Source: CAD feature listing. Evaluate the final solid. Frame: model axes, mm. A direction names the side the tool comes from. Round coordinates to 2 decimals unless told otherwise and drop trailing zeros. Write each question's results on one line, items separated by ' | '. Start each with the question number.
1. Ray query, line 1 (Y direction, x = 0, z = -4.25) (3 decimals); line 2 (Y direction, x = 0, z = 15) (3 decimals); line 3 (X direction, y = 40.5, z = 4.5). Return the intervals inside material, ascending.
2. Section A-A on z = -14.5. Give the number of separate pieces and of enclosed holes in the cut face, and give its area (3 significant figures).
3. Draft query along X for faces 3 (the flat face through (-17, -51, -20.638)), 4 (the cylindrical face through (40.8, -18.1, 5.5)). Return one class per face: released by +X, released by -X, zero draft, split by the parting line, or undercut.
4. Set-up query: faces 1 (the cylindrical face through (-11.43, -51.45, 15.94)), 2 (the cylindrical face through (7.363, 43.945, 5.529)). Return all of +Z, -Z, +X, -X, +Y, -Y with unobstructed straight access to the full face (end or side cutting, diameter ignored); none if empty.
5. Contact query for flat-ended pins moving along their axis: pin 1 Ø5 at (x, z) = (16.5, -9.5) entering from +Y; pin 2 Ø10 at (x, y) = (35.5, -36.5) entering from -Z; pin 3 Ø3 at (x, z) = (-23.5, 7) entering from -Y. Output: stop coordinate, or through.
Autodesk Inventor part; units mm, degrees
ref_plane "Work Plane1" through (0, 0, 0) normal (0, 0, 1) x (1, 0, 0)
ref_plane "YZ Plane" through (0, 0, 0) normal (1, 0, 0) x (0, 1, 0)
ref_plane "XZ Plane" through (0, 0, 0) normal (0, 1, 0) x (-1, 0, 0)
sketch "Sketch1" plane through (0, 0, 0) normal (0, 0, 1) x (1, 0, 0)
  circle A0 centre (0, 0) radius 55.88
  circle A1 centre (0, 0) radius 9.525
  line L0 (7.391, 0) -> (3.6955, -6.4008)
  line L1 (3.6955, -6.4008) -> (-3.6955, -6.4008)
  line L2 (-3.6955, -6.4008) -> (-7.391, 0)
  line L3 (-7.391, 0) -> (-3.6955, 6.4008)
  line L4 (-3.6955, 6.4008) -> (3.6955, 6.4008)
  line L5 (3.6955, 6.4008) -> (7.391, 0)
  circle A2 centre (0, 0) radius 52.705
  point P0 (0, 9.525)
  dimension "d1" = 19.05
  dimension "d0" = 111.76
  dimension "d2" = 12.8016
  dimension "d3" = 3.175
extrude "Extrusion1" add sketch "Sketch1" along normal mid plane 41.275 contours A0 | A1 | A2
sketch "Sketch4" plane through (0, 0, 20.6375) normal (0, 0, 1) x (1, 0, 0)
  circle A0 centre (0, 0) radius 52.705
  circle A1 centre (0, 0) radius 55.88 construction
  dimension "d59" = 3.175
extrude "Extrusion4" cut sketch "Sketch4" against normal blind 12.7
sketch "Sketch5" plane through (0, 0, -20.6375) normal (0, 0, -1) x (-1, 0, 0)
  circle A0 centre (0, 0) radius 9.525
  line L0 (3.6955, 6.4008) -> (7.391, 0)
  line L1 (7.391, 0) -> (3.6955, -6.4008)
  line L2 (3.6955, -6.4008) -> (-3.6955, -6.4008)
  line L3 (-3.6955, -6.4008) -> (-7.391, 0)
  line L4 (-7.391, 0) -> (-3.6955, 6.4008)
  line L5 (-3.6955, 6.4008) -> (3.6955, 6.4008)
  line L6 (3.6955, 6.4008) -> (7.391, 0)
  dimension "d26" = 19.05
extrude "Extrusion5" add sketch "Sketch5" along normal blind 3.175
sketch "Sketch6" plane through (0, 0, -20.6375) normal (0, 0, -1) x (-1, 0, 0)
  circle A0 centre (0, 0) radius 52.705
  circle A1 centre (0, 0) radius 9.525
  circle A2 centre (0, 0) radius 55.88 construction
  dimension "d60" = 3.175
extrude "Extrusion6" cut sketch "Sketch6" against normal blind 23.8252
sketch "Sketch7" plane through (0, 0, 7.9375) normal (0, 0, 1) x (1, 0, 0)
  circle A0 centre (0, 0) radius 9.525
  circle A1 centre (0, 0) radius 52.705
  circle A2 centre (0, 0) radius 47.9425 construction
  circle A3 centre (0, 0) radius 14.2875 construction
  line L0 (-9.7714, 10.4237) -> (-9.7714, 46.9362) construction
  line L1 (-9.7714, 10.4237) -> (16.8454, 44.8856)
  line L2 (-9.7714, 10.4237) -> (-36.3881, 44.8856)
  arc A4 (16.8454, 44.8856) -> (-36.3881, 44.8856) centre (-9.7714, -126.8345) ccw
  point P0 (-6.5143, 6.9491)
  dimension "d42" = 4.7625
  dimension "d41" = 4.7625
  dimension "d43" = 34.4619
  dimension "d44" = 36.5125
  dimension "d45" = 4.7625
extrude "Extrusion8" [suppressed]
fillet "Fillet1" [suppressed]
pattern_circular "Circular Pattern1" [suppressed]
fillet "Fillet2" [suppressed]
sketch "Sketch8" plane through (0, 0, 20.6375) normal (0, 0, 1) x (1, 0, 0)
  circle A0 centre (0, 0) radius 55.88
  circle A1 centre (0, 0) radius 57.15
  dimension "d53" = 114.3
extrude "Extrusion9" add sketch "Sketch8" against normal blind 1.5875
ref_plane "Work Plane1" through (0, 0, 0) normal (0, 0, 1) x (1, 0, 0)
mirror "Mirror1" about plane through (0, 0, 0) normal (0, 0, 1) of "Extrusion9"
fillet "Fillet3" radius 3.175 1 edges at (9.525, 0, 3.1877)
fillet "Fillet4" radius 3.175 1 edges at (-52.705, 0, 7.9375)
fillet "Fillet5" radius 3.175 1 edges at (52.705, 0, 3.1877)
sketch "Sketch9" plane through (0, 0, 3.1877) normal (0, 0, -1) x (-1, 0, 0)
  circle A0 centre (0, 0) radius 12.7 construction
  circle A1 centre (0, 0) radius 49.53 construction
  circle A2 centre (0, 0) radius 12.7 construction
  line L0 (0, -12.7) -> (0, -17.78) construction
  arc A3 (3.0152, -16.7853) -> (-3.1007, -17.0973) centre (0, -17.78) ccw
  circle A4 centre (0, 0) radius 49.53 construction
  line L1 (3.0152, -16.7853) -> (10.9727, -40.9066)
  line L2 (-3.1007, -17.0973) -> (-8.5623, -41.9032)
  arc A5 (8.941, -44.8445) -> (10.9502, -40.8384) centre (7.935, -41.8331) ccw
  arc A6 (-8.4774, -41.5179) -> (-6.215, -45.2629) centre (-5.3767, -42.2006) ccw
  arc A7 (-6.215, -45.2629) -> (8.941, -44.8445) centre (0.674, -20.0971) ccw
  point P0 (-10.4488, -48.4153)
  point P1 (10.4488, -48.4153)
  dimension "d62" = 5.08
  dimension "d63" = 6.35
  dimension "d77" = 25.4
  dimension "d78" = 25.4
  dimension "d79" = 6.35
  dimension "d80" = 6.35
  dimension "d81" = 13.3117
  dimension "d82" = 24.0531
  dimension "d83" = 42.2006
  dimension "d84" = 26.0917
  dimension "d85" = 17.78
extrude "Extrusion10" cut sketch "Sketch9" against normal up to next
pattern_circular "Circular Pattern2" count 9 over 360 about axis through (0, 0, -20.6375) along (0, 0, -1) of "Extrusion10"
properties part number "Custom Wheel" material "Aluminum 6061"
Taken from the geometry:
1) line 1: -55.88 to -52.705, -9.525 to -6.401, 6.401 to 9.525, 52.705 to 55.88 | line 2: -55.88 to -52.705, 52.705 to 55.88 | line 3: -38.5 to -21.19, -3.63 to 6.05, 21.77 to 38.5
2) separate pieces: 2 | enclosed holes: 2 | area: 1,230 mm^2
3) face 3: zero draft | face 4: undercut
4) face 1: +Z | face 2: +Z, -Z
5) pin 1: y = 54.1 | pin 2: z = -20.64 | pin 3: y = -51.37
